The model under review builds one solid part; all positions refer to its coordinate system, in mm. A direction names the side the tool comes from. Give positions to 0.01 mm unless a question says otherwise; leave off trailing zeros. Loops run counter-clockwise (first coordinate to the right, second up) from the corner with the lowest first, then second, coordinate; pieces in that order, holes last. Notation, with made-up numbers: M 22,63 L 36,63 A27 ccw 36,79 Z; hole C 61.5,-39 d7. An arc over 180 degrees is marked long. Put each result on its own line as item: value. Start each with the question number.
```python
from build123d import *

# Parameters (mm, degrees)
F0_R     = 9
F0_R_2   = 8
F1_DEPTH = 2
F0_R_3   = 7
F2_DEPTH = 5
F0_R_4   = 25
F3_DEPTH = 30


with BuildPart() as f1:
    # F0 (on Top) → F1 (new body)
    with BuildSketch(Plane.XY):
        with BuildLine():
            ThreePointArc((-19.918584, -11.5), (5.952838, -22.216294), (23, 0))
            ThreePointArc((23, 0), (5.952838, 22.216294), (-19.918584, 11.5))
            Line((-19.918584, 11.5), (-18.186533, 10.5))
            Line((-18.186533, 10.5), (-8.660254, 5))
            ThreePointArc((-8.660254, 5), (-10, 0), (-8.660254, -5))
            Line((-8.660254, -5), (-18.186533, -10.5))
            Line((-18.186533, -10.5), (-19.918584, -11.5))
        make_face()
        Circle(F0_R, mode=Mode.SUBTRACT)
        Circle(F0_R)
        Circle(F0_R_2, mode=Mode.SUBTRACT)
        with BuildLine():
            Line((-18.186533, 10.5), (-19.918584, 11.5))
            ThreePointArc((-19.918584, 11.5), (-23, 0), (-19.918584, -11.5))
            Line((-19.918584, -11.5), (-18.186533, -10.5))
            ThreePointArc((-18.186533, -10.5), (-21, 0), (-18.186533, 10.5))
        make_face()
    extrude(amount=F1_DEPTH)

    # F0 (on Top) → F2 (join)
    with BuildSketch(Plane.XY):
        Circle(F0_R_2)
        Circle(F0_R_3, mode=Mode.SUBTRACT)
    extrude(amount=F2_DEPTH)

    # F0 (on Top) → F3 (join)
    with BuildSketch(Plane.XY):
        Circle(F0_R_4)
        with BuildLine():
            ThreePointArc((-19.918584, 11.5), (5.952838, 22.216294), (23, 0))
            ThreePointArc((23, 0), (5.952838, -22.216294), (-19.918584, -11.5))
            ThreePointArc((-19.918584, -11.5), (-23, 0), (-19.918584, 11.5))
        make_face(mode=Mode.SUBTRACT)
    extrude(amount=F3_DEPTH)


solid = f1.part
```
Item 1: Consider section C-C, the plane y = 14. Write out the cut boundary in (x, z), plus the area to 3 significant figures.
Item 2: To check wall thickness, follow L1, parallel to Y at x = 0, z = 2.05; L2, parallel to Z at x = 20, y = 10.5; L3, parallel to X at y = 3.5, z = 3.5. State the ranges of each line that lie inside material, in increasing order. Write a range as [from, to].
Item 3: Consider section D-D, the plane y = 22. Write out the cut boundary in (x, z).
Item 4: Clearance check with flat-ended pins moving along their axes: pin 1 Ø10 at (x, y) = (-4, 0) entering from +Z; pin 2 Ø2 at (x, y) = (-10, -10.5) entering from +Z; pin 3 Ø3 at (x, y) = (-3.5, 0) entering from -Z; pin 4 Ø10 at (y, z) = (9.5, 17.5) entering from -X. State where each tip first meets the part, or that it passes through.
Item 5: Consider section A-A, the plane x = 0. Write out the cut boundary in (y, z).
Item 6: Draft analysis for pull direction Y (two halves, no side actions). For faces 4 (the cylindrical face through (23.846, 7.509, 14.79)), 5 (the cylindrical face through (-10, 0, 1)), 6 (the flat face through (22.1, -7.3, 30)), state which applies: +Y half, -Y half, draft (parallel to the pull), parting line (faces both ways), or undercut.
Item 7: Consider section B-B, the plane z = 19.5. Write out the cut boundary in (x, y), plus the area to 3 significant figures.
Item 8: Tool access review of faces 1 (the cylindrical face through (-1.73, -7.81, 3.48)), 2 (the flat face through (-13.49, 7.79, 0.99)), 3 (the flat face through (5.2, -5.2, 0)): name each direction out of +Z, -Z, +X, -X, +Y, -Y from which nothing blocks a thin tool from reaching the whole face with its end or side.
Report:
1. outline: M -20.71,0 L 20.71,0 L 20.71,30 L 18.25,30 L 18.25,2 L -18.25,2 L -18.25,30 L -20.71,30 Z
1. area: 221 mm²
2. L1: [-25, -23], [-8, -7], [7, 8], [23, 25]
2. L2: [0, 2]
2. L3: [-24.75, -22.73], [-7.19, -6.06], [6.06, 7.19], [22.73, 24.75]
3. outline: M -11.87,0 L 11.87,0 L 11.87,30 L 6.71,30 L 6.71,2 L -6.71,2 L -6.71,30 L -11.87,30 Z
4. pin 1: z = 5
4. pin 2: z = 2
4. pin 3: through
4. pin 4: x = -24.59
5. outline: M -25,0 L -7,0 L -7,5 L -8,5 L -8,2 L -23,2 L -23,30 L -25,30 Z; M 7,0 L 25,0 L 25,30 L 23,30 L 23,2 L 8,2 L 8,5 L 7,5 Z
6. face 4: parting line
6. face 5: undercut
6. face 6: draft
7. outline: C 0,0 d50; hole M -19.92,-11.5 A23 ccw long -19.92,11.5 A23 ccw Z
7. area: 302 mm²
8. face 1: +Z
8. face 2: +Z, -Z
8. face 3: -Z, +X, -X, +Y, -Y
